The figure shows three views and two pictorial views of one solid part (mm, origin at its lowest corner). Answer the questions. Round coordinates to 2 decimals unless told otherwise and drop trailing zeros. Write each loop counter-clockwise with the first axis right and the second up, starting at its lowest first coordinate (ties: lowest second). Pieces come first, ordered by that corner, then holes. Notation, with made-up numbers: (83, 17) -> (138, 17) arc R11 ccw to (138, 26) -> close; hole circle Ø6 at (58, 59). An arc over 180 degrees is marked (long way). One line per item, written item: value.
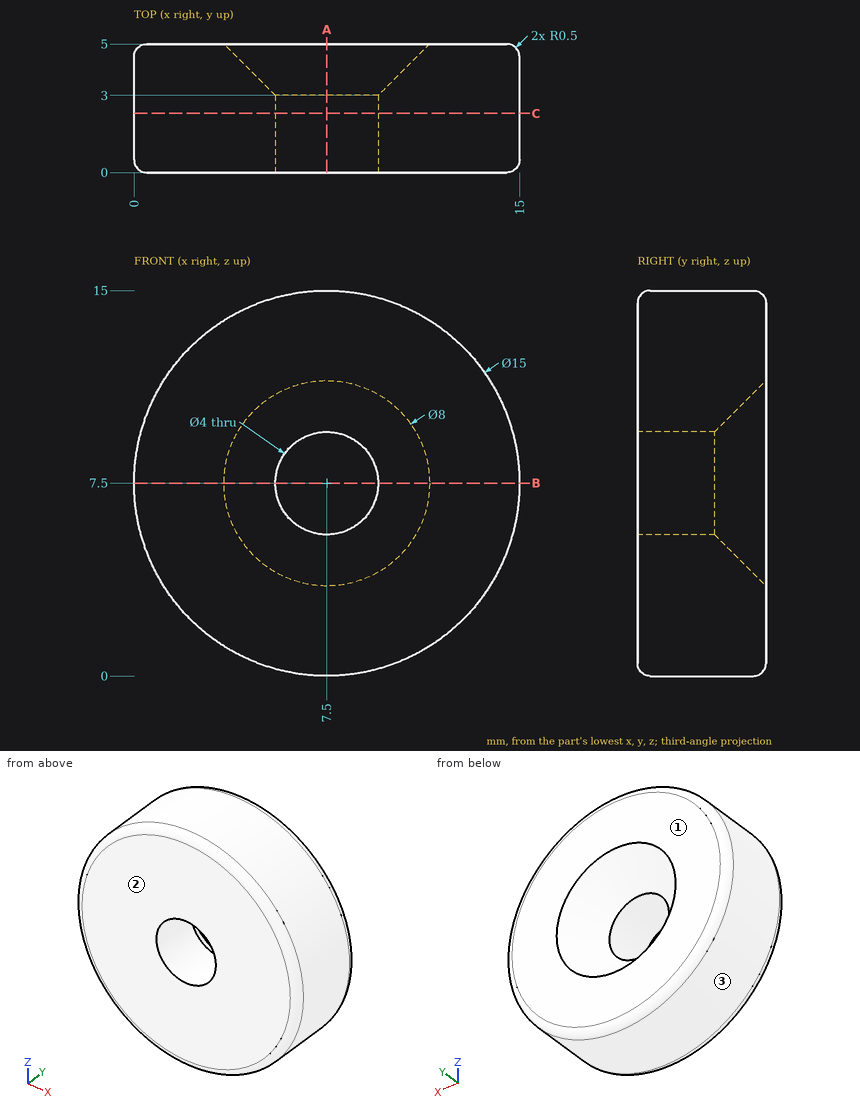
(1) For a pull along Y with two mould halves and no side action, classify the marked faces 1, 2 and 3 as pulls with the +Y half, pulls with the -Y half, needs draft (parallel to the pull), parting line crosses it, or undercut.
Reported:
face 1: pulls with the +Y half
face 2: pulls with the -Y half
face 3: needs draft
(2) Consider probe 1 along Z at (x, y) = (7.5, 0.7); probe 2 along X at (y, z) = (1.8, 5.75). Determine where each line is inside the solid, lowest interval first.
Reported:
probe 1: z = 0 to 5.5, 9.5 to 15
probe 2: x = 0.21 to 6.53, 8.47 to 14.79
(3) Find section C-C on y = 2.3. Give the vertices of the cut face in (x, z), plus the area to 3 significant figures.
Reported:
outline: circle Ø15 at (7.5, 7.5); hole circle Ø4 at (7.5, 7.5)
area: 164 mm2
(4) Flat-ended cylindrical pins translate along their axes: pin 1 Ø1.5 at (x, z) = (5, 6.5) entering from -Y; pin 2 Ø2 at (x, y) = (9, 2.5) entering from +Z. Find the tip coordinate at first contact, or state that the pin passes through.
Reported:
pin 1: stops at y = 0
pin 2: stops at z = 14.98
(5) Find section A-A on x = 7.5. Give the vertices of the cut face in (y, z), plus the area to 3 significant figures.
Reported:
outline: (0, 0.5) arc R0.5 ccw to (0.5, 0) -> (4.5, 0) arc R0.5 ccw to (5, 0.5) -> (5, 3.5) -> (3, 5.5) -> (0, 5.5) -> close; (0, 9.5) -> (3, 9.5) -> (5, 11.5) -> (5, 14.5) arc R0.5 ccw to (4.5, 15) -> (0.5, 15) arc R0.5 ccw to (0, 14.5) -> close
area: 50.8 mm2
(6) Find section B-B on z = 7.5. Give the vertices of the cut face in (x, y), plus the area to 3 significant figures.
Reported:
outline: (0, 0.5) arc R0.5 ccw to (0.5, 0) -> (5.5, 0) -> (5.5, 3) -> (3.5, 5) -> (0.5, 5) arc R0.5 ccw to (0, 4.5) -> close; (9.5, 0) -> (14.5, 0) arc R0.5 ccw to (15, 0.5) -> (15, 4.5) arc R0.5 ccw to (14.5, 5) -> (11.5, 5) -> (9.5, 3) -> close
area: 50.8 mm2
